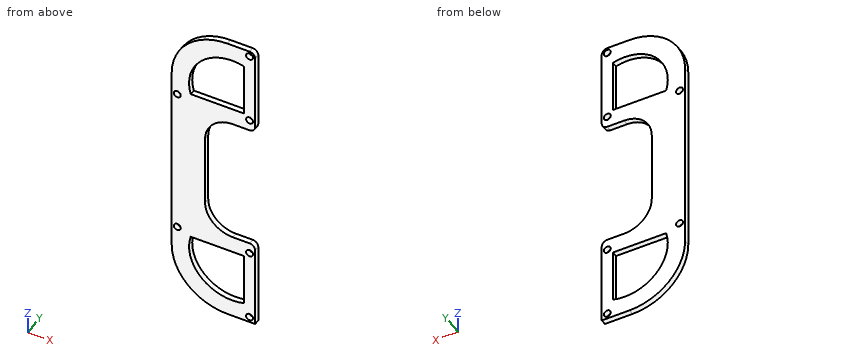
from build123d import *

# Parameters (mm, degrees)
SKETCH_1_W          = 30
SKETCH_1_H          = 110
EXTRUDE_1_DEPTH     = 2
SKETCH_2_R          = 1.25
CUT_EXTRUDE_1_DEPTH = 2
FILLET_1_R          = 20
FILLET_2_R          = 2
SKETCH_3_W          = 18
SKETCH_3_H          = 46
CUT_EXTRUDE_2_DEPTH = 2
FILLET_4_R          = 10
FILLET_5_R          = 2
CUT_EXTRUDE_3_DEPTH = 10


with BuildPart() as part:
    # 草图1 → 凸台-拉伸1 (new body)
    with BuildSketch(Plane(origin=(0, 0, 0), x_dir=(1, 0, 0), z_dir=(0, 1, 0))):
        Rectangle(SKETCH_1_W, SKETCH_1_H)
    extrude(amount=EXTRUDE_1_DEPTH)

    # 草图2 → 切除-拉伸1 (cut)
    with BuildSketch(Plane(origin=(0, 2, 0), x_dir=(1, 0, 0), z_dir=(0, 1, 0))):
        with Locations(Location((13, 27, 0), (0, 0, 270))):
            Circle(SKETCH_2_R)
        with Locations(Location((-13, 27, 0), (0, 0, 90))):
            Circle(SKETCH_2_R)
        with Locations(Location((13, 53, 0), (0, 0, 270))):
            Circle(SKETCH_2_R)
        with Locations(Location((13, -53, 0), (0, 0, 90))):
            Circle(SKETCH_2_R)
        with Locations(Location((-13, -27, 0), (0, 0, 270))):
            Circle(SKETCH_2_R)
        with Locations(Location((13, -27, 0), (0, 0, 90))):
            Circle(SKETCH_2_R)
    extrude(amount=-CUT_EXTRUDE_1_DEPTH, mode=Mode.SUBTRACT)

    # 圆角1
    fillet_1_edges = [part.edges().sort_by_distance(p)[0] for p in [
        (-15, 1, 55),
        (-15, 1, -55),
    ]]
    fillet(fillet_1_edges, radius=FILLET_1_R)

    # 圆角2
    fillet_2_edges = [part.edges().sort_by_distance(p)[0] for p in [
        (15, 1, 55),
    ]]
    fillet(fillet_2_edges, radius=FILLET_2_R)

    # 草图3 → 切除-拉伸2 (cut)
    with BuildSketch(Plane(origin=(0, 2, 0), x_dir=(1, 0, 0), z_dir=(0, 1, 0))):
        with Locations((6, 0)):
            Rectangle(SKETCH_3_W, SKETCH_3_H)
    extrude(amount=-CUT_EXTRUDE_2_DEPTH, mode=Mode.SUBTRACT)

    # 圆角4
    fillet_4_edges = [part.edges().sort_by_distance(p)[0] for p in [
        (-3, 1, -23),
        (-3, 1, 23),
    ]]
    fillet(fillet_4_edges, radius=FILLET_4_R)

    # 圆角5
    fillet_5_edges = [part.edges().sort_by_distance(p)[0] for p in [
        (15, 1, -23),
        (15, 1, 23),
    ]]
    fillet(fillet_5_edges, radius=FILLET_5_R)

    # 草图4 → 切除-拉伸3 (cut)
    with BuildSketch(Plane(origin=(0, 2, 0), x_dir=(1, 0, 0), z_dir=(0, 1, 0))):
        with BuildLine():
            Line((11, 48.171572875), (11, 29))
            Line((11, 29), (-8.171572875, 29))
            ThreePointArc((-8.171572875, 29), (-4.228384219, 44.228384219), (11, 48.171572875))
        make_face()
        with BuildLine():
            Line((11, -29), (-8.171572875, -29))
            ThreePointArc((-8.171572875, -29), (-4.228384219, -44.228384219), (11, -48.171572875))
            Line((11, -48.171572875), (11, -29))
        make_face()
    extrude(amount=-CUT_EXTRUDE_3_DEPTH, mode=Mode.SUBTRACT)


solid = part.part
The listing builds one solid part. Answer for the finished solid, in the listing's coordinates (mm). Give positions to 0.01 mm unless a question says otherwise; leave off trailing zeros. Order: outer loops, then holes, each group sorted by start corner. A loop starts at its lowest first (then second) coordinate and runs counter-clockwise, first axis right, second up. Notation, with made-up numbers: (-21.5, 77.25) - (7.5, 77.25) arc R15 ccw to (7.5, 95.25) - close; hole circle Ø8 at (11, 87). An arc over 180 degrees is marked (long way). One line per item, written item: value. Start each with the question number.
1) Given pin 1 Ø0.6 at (x, y) = (3.5, 1) entering from -Z; pin 2 Ø0.6 at (y, z) = (1.5, -40) entering from -X, each flat-ended and moving along its own axis, determine where each tip first touches the part or whether it passes through.
2) A cutting plane is placed at D-D on z = 40.5. Give the vertices of the cut face in (x, y), then the cut area to 3 significant figures.
3) A cutting plane is placed at A-A on z = 27. Give the vertices of the cut face in (x, y).
4) Find the intervals of material crossed by L1, parallel to X at y = 1.25, z = -27; L2, parallel to Z at x = 7, y = 0.95; L3, parallel to Z at x = -1.5, y = 1.45, in increasing order.
5) A cutting plane is placed at C-C on x = 3.5. Give the vertices of the cut face in (y, z), then the cut area to 3 significant figures.
6) A cutting plane is placed at B-B on y = 1.45. State how many separate pieces and enclosed holes the cut face has, then the cut area to 3 significant figures.
Answer sheet:
1. pin 1: stops at z = -54.96
1. pin 2: stops at x = -14.44
2. outline: (-14.23, 0) - (-6.98, 0) - (-6.98, 2) - (-14.23, 2) - close; (11, 0) - (15, 0) - (15, 2) - (11, 2) - close
2. area: 22.5 mm2
3. outline: (-15, 0) - (-14.25, 0) - (-14.25, 2) - (-15, 2) - close; (-11.75, 0) - (11.75, 0) - (11.75, 2) - (-11.75, 2) - close; (14.25, 0) - (15, 0) - (15, 2) - (14.25, 2) - close
4. L1: x = -15 to -14.25, -11.75 to 11.75, 14.25 to 15
4. L2: z = -55 to -48.77, -29 to -23, 23 to 29, 48.77 to 55
4. L3: z = -53.91 to -46.4, -29 to -18.27, 18.27 to 29, 46.4 to 53.91
5. outline: (0, -54.94) - (2, -54.94) - (2, -48.43) - (0, -48.43) - close; (0, -29) - (2, -29) - (2, -22.37) - (0, -22.37) - close; (0, 22.37) - (2, 22.37) - (2, 29) - (0, 29) - close; (0, 48.43) - (2, 48.43) - (2, 54.94) - (0, 54.94) - close
5. area: 52.6 mm2
6. separate pieces: 1
6. enclosed holes: 8
6. area: 1,640 mm2
